The figure shows three views and two pictorial views of one solid part (mm, origin at its lowest corner). Answer the questions. A direction names the side the tool comes from. Coordinates: 2 decimals unless noted, no trailing zeros. Loops run counter-clockwise (first coordinate to the right, second up) from the corner with the lowest first, then second, coordinate; pieces in that order, holes last. Notation, with made-up numbers: (78, 36) - (107, 36) arc R5 cw to (107, 42) - close; hole circle Ø4 at (25.25, 29). An arc over 180 degrees is marked (long way). Return JSON: item names as keys, results as strings. Group by question number.
1. Which of the six approach directions +Z, -Z, +X, -X, +Y, -Y give full straight-line access (tool end or side, diameter ignored) to the marked faces 1 and 2?
2. Section B-B (y = 122) is taken. Write down the section's boundary in (x, z) (1 decimal), and give its area (3 significant figures).
3. The mould has two halves that part along Y. Classify the marked faces 3, 4 and 5: pulls with the +Y half, pulls with the -Y half, needs draft (parallel to the pull), parting line crosses it, or undercut.
4. Section C-C (z = 83) is taken. Write down the section's boundary in (x, y) (1 decimal).
5. Each of these flat-tipped pins is pushed along its axis until it touches: P1, Ø13.5, axis at x = 91.5, y = 142, coming from the +Z side; P2, Ø14.5, axis at y = 73.09, z = 57.53, coming from the -X side. Where does it stop, or does it pass through?
6. Find the intervals of material crossed by line 1 along X through (y, z) = (117, 54) (1 decimal); line 2 along Y through (x, z) = (112.5, 35.5), in increasing order.
7. Section A-A (x = 96) is taken. Write down the section's boundary in (y, z), and give its area (3 significant figures).
8. Section D-D (z = 7) is taken. Write down the section's boundary in (x, y) (1 decimal), and give its area (3 significant figures).
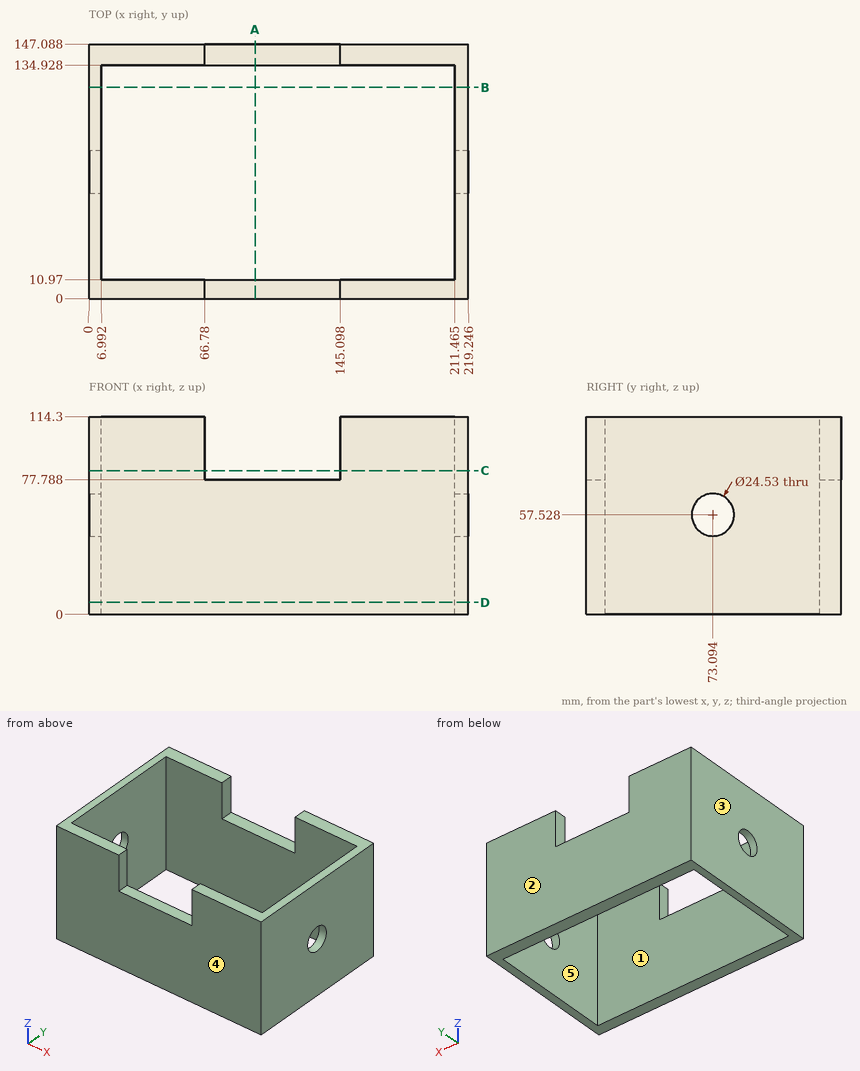
The answers:
{
 "1": {"face 1": "+Z, -Z", "face 2": "+Z, -Z, +X, -X, +Y"},
 "2": {"outline": "(0, 0) - (7, 0) - (7, 114.3) - (0, 114.3) - close; (211.5, 0) - (219.2, 0) - (219.2, 114.3) - (211.5, 114.3) - close", "area": "1,690 mm2"},
 "3": {"face 3": "needs draft", "face 4": "pulls with the -Y half", "face 5": "undercut"},
 "4": {"outline": "(0, 0) - (66.8, 0) - (66.8, 11) - (7, 11) - (7, 134.9) - (66.8, 134.9) - (66.8, 147.1) - (0, 147.1) - close; (145.1, 0) - (219.2, 0) - (219.2, 147.1) - (145.1, 147.1) - (145.1, 134.9) - (211.5, 134.9) - (211.5, 11) - (145.1, 11) - close"},
 "5": {"P1": "stops at z = 77.79", "P2": "passes through"},
 "6": {"line 1": "x = 0 to 7, 211.5 to 219.2", "line 2": "y = 0 to 10.97, 134.93 to 147.09"},
 "7": {"outline": "(0, 0) - (10.97, 0) - (10.97, 77.79) - (0, 77.79) - close; (134.93, 0) - (147.09, 0) - (147.09, 77.79) - (134.93, 77.79) - close", "area": "1,800 mm2"},
 "8": {"outline": "(0, 0) - (219.2, 0) - (219.2, 147.1) - (0, 147.1) - close; hole (7, 11) - (211.5, 11) - (211.5, 134.9) - (7, 134.9) - close", "area": "6,900 mm2"}
}
